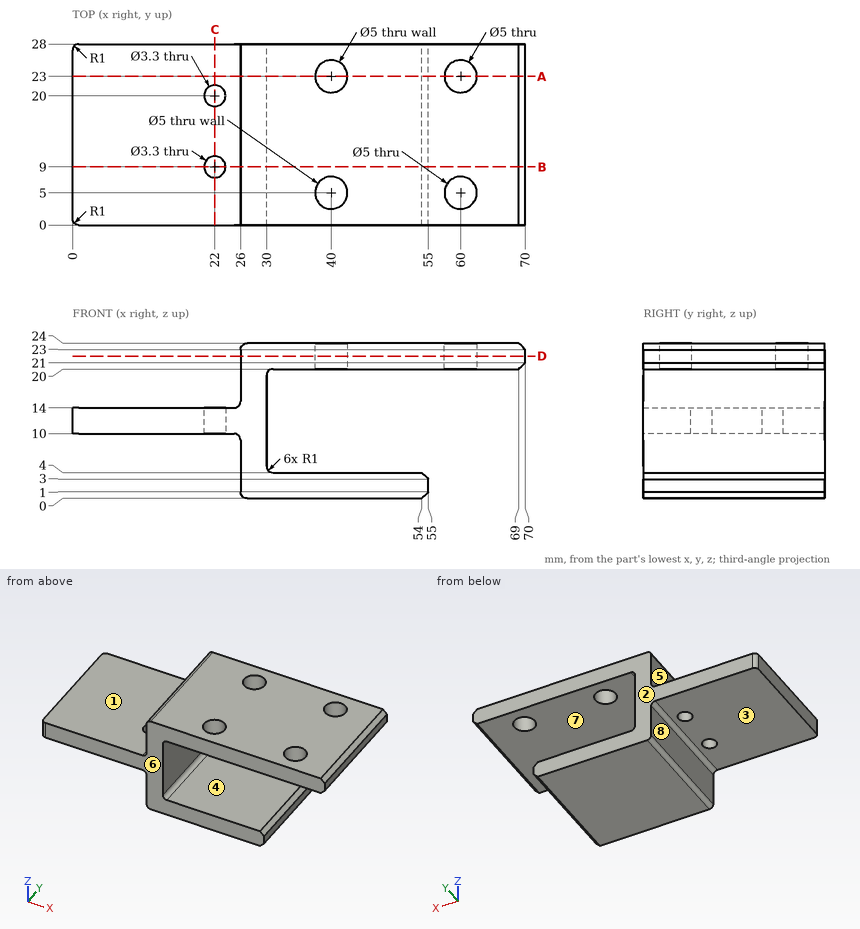
Job drawing, mm, ordinate dimensions from the low corner. One solid piece. A direction names the side the tool comes from. Round coordinates to 2 decimals unless told otherwise and drop trailing zeros. Loops run counter-clockwise (first coordinate to the right, second up) from the corner with the lowest first, then second, coordinate; pieces in that order, holes last. Notation, with made-up numbers: M -21,14.5 L 17,14.5 A21 ccw 17,35.5 Z; hole C 5,75.5 d9. An arc over 180 degrees is marked long. One line per question, with ' | ' between items. Start each with the question number.
Item 1: Cut at C-C, the plane x = 22. Write the cut outline in (y, z).
Item 2: Cut at A-A, the plane y = 23. State how many separate pieces and enclosed holes the cut face has, plus the area to 3 significant figures.
Item 3: Pin check, flat tips, straight feed: pin 1 Ø4 at (x, y) = (22, 20) entering from -Z; pin 2 Ø12 at (y, z) = (21, 21) entering from -X; pin 3 Ø4.5 at (x, y) = (40, 5) entering from +Z. Stop position of each tip, or through.
Item 4: Which spindle directions (+Z, -Z, +X, -X, +Y, -Y) get a long thin tool onto all of the face, cutting with end or side? Do the marked faces 5, 6, 7 and 8. Say none if no direction does.
Item 5: Wall check: line 1 (Y direction, x = 60, z = 21.35); line 2 (Z direction, x = 36, y = 5); line 3 (X direction, y = 2.25, z = 13.75). Give the ranges that are in metal, low to high.
Item 6: Cut at B-B, the plane y = 9. Write the cut outline in (x, z).
Item 7: Two-plate mould, pull along Z, no slides. Class the marked faces 1, 2, 3 and 4: pulls with the +Z half, pulls with the -Z half, needs draft (parallel to the pull), parting line crosses it, or undercut.
Item 8: Cut at D-D, the plane z = 22. Write the cut outline in (x, y), plus the area to 3 significant figures.
Responses:
1) outline: M 0,10 L 7.35,10 L 7.35,14 L 0,14 Z; M 10.65,10 L 18.35,10 L 18.35,14 L 10.65,14 Z; M 21.65,10 L 28,10 L 28,14 L 21.65,14 Z
2) separate pieces: 3 | enclosed holes: 0 | area: 418 mm²
3) pin 1: stops at z = 10 | pin 2: stops at x = 26 | pin 3: stops at z = 4
4) face 5: +Z, -X, +Y, -Y | face 6: +Z, -Z, +X, -X, -Y | face 7: +X, +Y, -Y | face 8: -Z, -X, +Y, -Y
5) line 1: y = 0 to 2.5, 7.5 to 20.5, 25.5 to 28 | line 2: z = 0 to 4, 20 to 24 | line 3: x = 0 to 30
6) outline: M 0,10 L 20.35,10 L 20.35,14 L 0,14 Z; M 23.65,10 L 25,10 A1 cw 26,9 L 26,1 A1 ccw 27,0 L 54,0 L 55,1 L 55,3 L 54,4 L 31,4 A1 cw 30,5 L 30,19 A1 cw 31,20 L 69,20 L 70,21 L 70,23 L 69,24 L 27,24 A1 ccw 26,23 L 26,15 A1 cw 25,14 L 23.65,14 Z
7) face 1: pulls with the +Z half | face 2: needs draft | face 3: pulls with the -Z half | face 4: undercut
8) outline: M 26,0 L 70,0 L 70,28 L 26,28 Z; hole C 40,5 d5; hole C 40,23 d5; hole C 60,5 d5; hole C 60,23 d5 | area: 1,150 mm²
